from build123d import *

# Parameters (mm, degrees)
BOSS_EXTRUDE1_DEPTH = 1
SKETCH2_R           = 3.5
BOSS_EXTRUDE2_DEPTH = 5
SKETCH3_R           = 2.0025
CUT_EXTRUDE1_DEPTH  = 7
CUT_EXTRUDE2_DEPTH  = 4


with BuildPart() as part:
    # Sketch1 → Boss-Extrude1 (new body)
    with BuildSketch(Plane(origin=(0, 0, 0), x_dir=(1, 0, 0), z_dir=(0, 1, 0))):
        with BuildLine():
            Line((-3.5, 4), (3.5, 4))
            ThreePointArc((3.5, 4), (7.5, 0), (3.5, -4))
            Line((3.5, -4), (-3.5, -4))
            ThreePointArc((-3.5, -4), (-7.5, 0), (-3.5, 4))
        make_face()
    extrude(amount=BOSS_EXTRUDE1_DEPTH)

    # Sketch2 → Boss-Extrude2 (add)
    with BuildSketch(Plane(origin=(0, 1, 0), x_dir=(1, 0, 0), z_dir=(0, 1, 0))):
        Circle(SKETCH2_R)
    extrude(amount=BOSS_EXTRUDE2_DEPTH)

    # Sketch3 → Cut-Extrude1 (cut, through all)
    with BuildSketch(Plane(origin=(0, 6, 0), x_dir=(1, 0, 0), z_dir=(0, 1, 0))):
        Circle(SKETCH3_R)
    extrude(amount=-CUT_EXTRUDE1_DEPTH, mode=Mode.SUBTRACT)

    # Sketch4 → Cut-Extrude2 (cut)
    with BuildSketch(Plane(origin=(0, 6, 0), x_dir=(1, 0, 0), z_dir=(0, 1, 0))):
        with BuildLine():
            Line((-1.856746146, 0.75), (-3.418698583, 0.75))
            ThreePointArc((-3.418698583, 0.75), (-3.5, 0), (-3.418698583, -0.75))
            Line((-3.418698583, -0.75), (-1.856746146, -0.75))
            ThreePointArc((-1.856746146, -0.75), (-2.0025, 0), (-1.856746146, 0.75))
        make_face()
        with BuildLine():
            ThreePointArc((3.418698583, -0.75), (3.5, 0), (3.418698583, 0.75))
            Line((3.418698583, 0.75), (1.856746146, 0.75))
            ThreePointArc((1.856746146, 0.75), (2.0025, 0), (1.856746146, -0.75))
            Line((1.856746146, -0.75), (3.418698583, -0.75))
        make_face()
    extrude(amount=-CUT_EXTRUDE2_DEPTH, mode=Mode.SUBTRACT)


solid = part.part
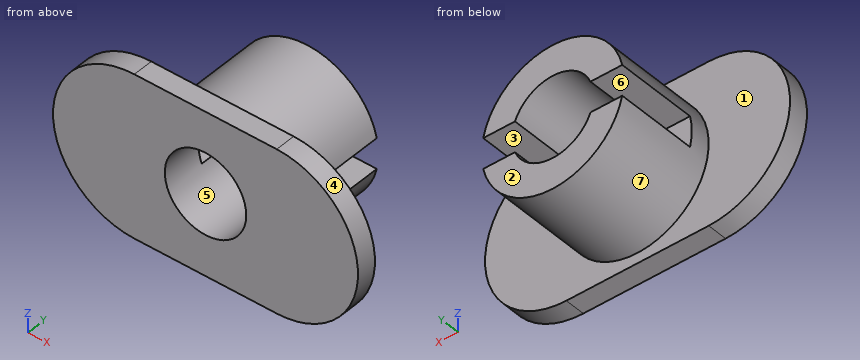
Could you check a few things on this model? Use its own coordinates, in mm. Face numbers are marked on the shaded views. A direction names the side the tool comes from. Coordinates: 2 decimals unless noted, no trailing zeros. Order: outer loops, then holes, each group sorted by start corner. A loop starts at its lowest first (then second) coordinate and runs counter-clockwise, first axis right, second up.
Q1. Will these pins go through, and if not, where does the flat tip stop? pin 1 (0.8 mm diameter, centred on x = 3, y = 4.5, fed in from -Z); pin 2 (1 mm diameter, centred on y = 1, z = 3, fed in from -X); pin 3 (1 mm diameter, centred on x = -5, z = 1, fed in from +Y).
Q2. Which directions (+Z, -Z, +X, -X, +Y, -Y) give clear straight access to the entire face, cutting with the end or side of a thin tool? Please do the marked faces 1, 2 and 3.
Q3. Suppose I cut it at D-D on z = 2.25. Please give me the cut outline in (x, y).
Q4. Suppose I cut it at A-A on x = 0. Please give me the cut outline in (y, z), and give its area (3 significant figures).
Q5. Thinking about a two-plate mould opening in X: for the marked faces 4, 5, 6 and 7, which applies, released by +X, released by -X, zero draft, split by the parting line, or undercut?
Q6. Suppose I cut it at C-C on z = 0. Please give me the cut outline in (x, y).
Q7. Please list where these lines run through material, in increasing order: L1, parallel to X at y = 1.5, z = 0; L2, parallel to X at y = 3.95, z = -1.25.
Answer:
1. pin 1: stops at z = -2.34
1. pin 2: stops at x = -6.62
1. pin 3: stops at y = 1
2. face 1: +Y
2. face 2: +Z, -Z, +X, -X, +Y
2. face 3: +X, -X, +Y
3. outline: (-6.81, 0) - (6.81, 0) - (6.81, 1) - (2.68, 1) - (2.68, 6) - (-2.68, 6) - (-2.68, 1) - (-6.81, 1) - close
4. outline: (0, -4) - (1, -4) - (1, -3.5) - (6, -3.5) - (6, -2) - (0, -2) - close; (0, 2) - (6, 2) - (6, 3.5) - (1, 3.5) - (1, 4) - (0, 4) - close
4. area: 19.0 mm2
5. face 4: released by +X
5. face 5: undercut
5. face 6: zero draft
5. face 7: split by the parting line
6. outline: (-7.5, 0) - (-2, 0) - (-2, 2) - (-3.5, 2) - (-3.5, 1) - (-7.5, 1) - close; (2, 0) - (7.5, 0) - (7.5, 1) - (3.5, 1) - (3.5, 2) - (2, 2) - close
7. L1: x = -3.5 to -2, 2 to 3.5
7. L2: x = -3.27 to -1.56, 1.56 to 3.27
